```python
from build123d import *

# Parameters (mm, degrees)
SKETCH1_W            = 126
SKETCH1_H            = 96
SKETCH1_R            = 1.675
BOSS_EXTRUDE1_DEPTH  = 1
SKETCH2_W            = 5
SKETCH2_H            = 10
BOSS_EXTRUDE2_DEPTH  = 12
CUT_EXTRUDE1_REACH   = 134.578
SKETCH3_R            = 1.675
CUT_EXTRUDE2_START   = -2
CUT_EXTRUDE2_DEPTH   = 114.5
CHAMFER1_SIZE        = 2
CUT_EXTRUDE3_REACH   = 134.578
SKETCH5_R            = 1.675
CUT_EXTRUDE4_START   = -2
CUT_EXTRUDE4_DEPTH   = 114.5
SKETCH7_R            = 1.675
CUT_EXTRUDE5_DEPTH   = 10
SKETCH9_W            = 7
SKETCH9_H            = 28
CUT_EXTRUDE7_DEPTH   = 10
SKETCH11_R           = 1.675
SKETCH11_W           = 9
SKETCH11_H           = 6
CUT_EXTRUDE8_DEPTH   = 10
BOSS_EXTRUDE3_DEPTH  = 2
SKETCH24_W           = 19
SKETCH24_H           = 25.6
CUT_EXTRUDE17_DEPTH  = 2
FILLET1_R            = 2
SKETCH26_W           = 42.95
SKETCH26_H           = 12.988932873
SKETCH26_W_2         = 30.05
SKETCH26_H_2         = 41.011067127
SKETCH26_H_3         = 28
BOSS_EXTRUDE10_DEPTH = 3
FILLET2_R            = 2


with BuildPart() as part:
    # Sketch1 → Boss-Extrude1 (new body)
    with BuildSketch(Plane.XY):
        Rectangle(SKETCH1_W, SKETCH1_H)
        with Locations((53, 31)):
            Circle(SKETCH1_R, mode=Mode.SUBTRACT)
        with Locations((53, 21)):
            Circle(SKETCH1_R, mode=Mode.SUBTRACT)
    extrude(amount=BOSS_EXTRUDE1_DEPTH)

    # Sketch2 → Boss-Extrude2 (add)
    with BuildSketch(Plane(origin=(0, 0, 0), x_dir=(-1, 0, 0), z_dir=(0, 0, -1))):
        with Locations((-57.5, 40)):
            Rectangle(SKETCH2_W, SKETCH2_H)
        with Locations((57.5, 40)):
            Rectangle(SKETCH2_W, SKETCH2_H)
        with Locations((-57.5, -40)):
            Rectangle(SKETCH2_W, SKETCH2_H)
        with Locations((57.5, -40)):
            Rectangle(SKETCH2_W, SKETCH2_H)
    extrude(amount=BOSS_EXTRUDE2_DEPTH)

    # Cut-Extrude1: up to this face of the body (flat: up to its plane)
    cut_extrude1_end = Plane(part.part.faces().sort_by_distance((60, 40, -6))[0])
    # Sketch3 → Cut-Extrude1 (cut, up to the picked face)
    with BuildSketch(Plane.ZY.offset(60), mode=Mode.PRIVATE) as cut_extrude1_sk1:
        with Locations((-7, 40)):
            Circle(SKETCH3_R)
    cut_extrude1_tool1 = split(extrude(cut_extrude1_sk1.sketch, amount=-CUT_EXTRUDE1_REACH, mode=Mode.PRIVATE), bisect_by=cut_extrude1_end, keep=Keep.BOTH, mode=Mode.PRIVATE)
    add(cut_extrude1_tool1.solids().sort_by(Axis((-60, 40, -7), (1, 0, 0)))[0], mode=Mode.SUBTRACT)

    # Sketch4 → Cut-Extrude2 (cut)
    with BuildSketch(Plane(origin=(-55, 0, 0), x_dir=(0, 0, -1), z_dir=(1, 0, 0)).offset(CUT_EXTRUDE2_START)):
        Polygon((8.616580754, 42.8), (5.383419246, 42.8), (3.766838493, 40), (5.383419246, 37.2), (8.616580754, 37.2), (10.233161507, 40), align=None)
    extrude(amount=CUT_EXTRUDE2_DEPTH, mode=Mode.SUBTRACT)

    # Chamfer1
    chamfer1_edges = [part.edges().sort_by_distance(p)[0] for p in [
        (55, 40, 0),
        (-55, 40, 0),
        (55, -40, 0),
        (-55, -40, 0),
    ]]
    chamfer(chamfer1_edges, length=CHAMFER1_SIZE)

    # Cut-Extrude3: up to this face of the body (flat: up to its plane)
    cut_extrude3_end = Plane(part.part.faces().sort_by_distance((-60, -40, -6))[0])
    # Sketch5 → Cut-Extrude3 (cut, up to the picked face)
    with BuildSketch(Plane(origin=(60, 0, 0), x_dir=(0, 0, -1), z_dir=(1, 0, 0)), mode=Mode.PRIVATE) as cut_extrude3_sk1:
        with Locations((7, -40)):
            Circle(SKETCH5_R)
    cut_extrude3_tool1 = split(extrude(cut_extrude3_sk1.sketch, amount=-CUT_EXTRUDE3_REACH, mode=Mode.PRIVATE), bisect_by=cut_extrude3_end, keep=Keep.BOTH, mode=Mode.PRIVATE)
    add(cut_extrude3_tool1.solids().sort_by(Axis((60, -40, -7), (-1, 0, 0)))[0], mode=Mode.SUBTRACT)

    # Sketch6 → Cut-Extrude4 (cut)
    with BuildSketch(Plane(origin=(-55, 0, 0), x_dir=(0, 0, -1), z_dir=(1, 0, 0)).offset(CUT_EXTRUDE4_START)):
        Polygon((8.616580754, -37.2), (5.383419246, -37.2), (3.766838493, -40), (5.383419246, -42.8), (8.616580754, -42.8), (10.233161507, -40), align=None)
    extrude(amount=CUT_EXTRUDE4_DEPTH, mode=Mode.SUBTRACT)

    # Sketch7 → Cut-Extrude5 (cut)
    with BuildSketch(Plane.XY.offset(1)):
        with Locations((5.63, 30)):
            Circle(SKETCH7_R)
        with Locations((-2.37, 30)):
            Circle(SKETCH7_R)
    extrude(amount=-CUT_EXTRUDE5_DEPTH, mode=Mode.SUBTRACT)

    # Sketch9 → Cut-Extrude7 (cut)
    with BuildSketch(Plane.XY.offset(1)):
        with Locations((-9.87, 29)):
            Rectangle(SKETCH9_W, SKETCH9_H)
    extrude(amount=-CUT_EXTRUDE7_DEPTH, mode=Mode.SUBTRACT)

    # Sketch11 → Cut-Extrude8 (cut)
    with BuildSketch(Plane.XY.offset(1)):
        with Locations((22, -36.45)):
            Circle(SKETCH11_R)
        with Locations((22, -22.45)):
            Circle(SKETCH11_R)
        with Locations((-12.5, -23.2)):
            Rectangle(SKETCH11_W, SKETCH11_H)
    extrude(amount=-CUT_EXTRUDE8_DEPTH, mode=Mode.SUBTRACT)

    # Sketch21 → Boss-Extrude3 (add)
    # profile 1 of 4: a face of its own
    with BuildSketch(Plane(origin=(0, 0, 0), x_dir=(-1, 0, 0), z_dir=(0, 0, -1))):
        Polygon((-50.719466437, 24.95), (-55.280533563, 24.95), (-57.561067127, 21), (-55.280533563, 17.05), (-50.719466437, 17.05), (-48.438932873, 21), align=None)
        Polygon((-51.397853003, 23.775), (-54.602146997, 23.775), (-56.204293994, 21), (-54.602146997, 18.225), (-51.397853003, 18.225), (-49.795706006, 21), align=None, mode=Mode.SUBTRACT)
    # profile 2 of 4: a face of its own
    with BuildSketch(Plane(origin=(0, 0, 0), x_dir=(-1, 0, 0), z_dir=(0, 0, -1))):
        Polygon((-50.719466437, 34.95), (-55.280533563, 34.95), (-57.561067127, 31), (-55.280533563, 27.05), (-50.719466437, 27.05), (-48.438932873, 31), align=None)
        Polygon((-51.397853003, 33.775), (-54.602146997, 33.775), (-56.204293994, 31), (-54.602146997, 28.225), (-51.397853003, 28.225), (-49.795706006, 31), align=None, mode=Mode.SUBTRACT)
    # profile 3 of 4: a face of its own
    with BuildSketch(Plane(origin=(0, 0, 0), x_dir=(-1, 0, 0), z_dir=(0, 0, -1))):
        Polygon((6.32, 32.280533563), (2.37, 34.561067127), (-1.58, 32.280533563), (-1.58, 27.719466437), (2.37, 25.438932873), (6.32, 27.719466437), align=None)
        Polygon((5.145, 31.602146997), (2.37, 33.204293994), (-0.405, 31.602146997), (-0.405, 28.397853003), (2.37, 26.795706006), (5.145, 28.397853003), align=None, mode=Mode.SUBTRACT)
    # profile 4 of 4: a face of its own
    with BuildSketch(Plane(origin=(0, 0, 0), x_dir=(-1, 0, 0), z_dir=(0, 0, -1))):
        Polygon((-1.68, 32.280533563), (-5.63, 34.561067127), (-9.58, 32.280533563), (-9.58, 27.719466437), (-5.63, 25.438932873), (-1.68, 27.719466437), align=None)
        Polygon((-2.855, 31.602146997), (-5.63, 33.204293994), (-8.405, 31.602146997), (-8.405, 28.397853003), (-5.63, 26.795706006), (-2.855, 28.397853003), align=None, mode=Mode.SUBTRACT)
    extrude(amount=BOSS_EXTRUDE3_DEPTH)

    # Sketch24 → Cut-Extrude17 (cut)
    with BuildSketch(Plane.XY.offset(1)):
        with Locations((-46.7, 1.15)):
            Rectangle(SKETCH24_W, SKETCH24_H)
        Polygon((-37.2, 26.35), (-37.2, 13.95), (-37.2, -11.65), (-37.2, -24.05), (-33.8, -24.05), (-33.8, 26.35), align=None)
    extrude(amount=-CUT_EXTRUDE17_DEPTH, mode=Mode.SUBTRACT)

    # Fillet1
    fillet1_edges = [part.edges().sort_by_distance(p)[0] for p in [
        (57.5, 45, -12),
        (57.5, 35, -12),
        (-57.5, 45, -12),
        (-57.5, 35, -12),
        (57.5, -35, -12),
        (57.5, -45, -12),
        (-57.5, -35, -12),
        (-57.5, -45, -12),
    ]]
    fillet(fillet1_edges, radius=FILLET1_R)

    # Sketch26 → Boss-Extrude10 (add)
    with BuildSketch(Plane(origin=(0, 0, 0), x_dir=(-1, 0, 0), z_dir=(0, 0, -1))):
        Polygon((-27.95, -30.011067127), (-27.95, -43), (-55, -43), (-55, -45), (55, -45), (55, -43), (19, -43), (19, -30.011067127), (58, -30.011067127), (58, -35), (60, -35), (60, 35), (58, 35), (58, 32), (19, 32), (19, 43), (60, 43), (60, 45), (-60, 45), (-60, 43), (-27.95, 43), (-27.95, 15), (-58, 15), (-58, 35), (-60, 35), (-60, -35), (-58, -35), (-58, -30.011067127), align=None)
        with Locations((-4.475, -36.505533564)):
            Rectangle(SKETCH26_W, SKETCH26_H, mode=Mode.SUBTRACT)
        with Locations((-42.975, -7.505533564)):
            Rectangle(SKETCH26_W_2, SKETCH26_H_2, mode=Mode.SUBTRACT)
        with Locations((-4.475, -7.505533564)):
            Rectangle(SKETCH26_W, SKETCH26_H_2, mode=Mode.SUBTRACT)
        with Locations((-4.475, 29)):
            Rectangle(SKETCH26_W, SKETCH26_H_3, mode=Mode.SUBTRACT)
        Polygon((19, 15), (19, 30), (58, 30), (58, -28.011067127), (19, -28.011067127), (19, 13), (33.8, 13), (33.8, 15), align=None, mode=Mode.SUBTRACT)
    extrude(amount=BOSS_EXTRUDE10_DEPTH)

    # Fillet2
    fillet2_edges = [part.edges().sort_by_distance(p)[0] for p in [
        (-63, 48, 0.5),
        (63, 48, 0.5),
        (63, -48, 0.5),
        (-63, -48, 0.5),
    ]]
    fillet(fillet2_edges, radius=FILLET2_R)


solid = part.part
```
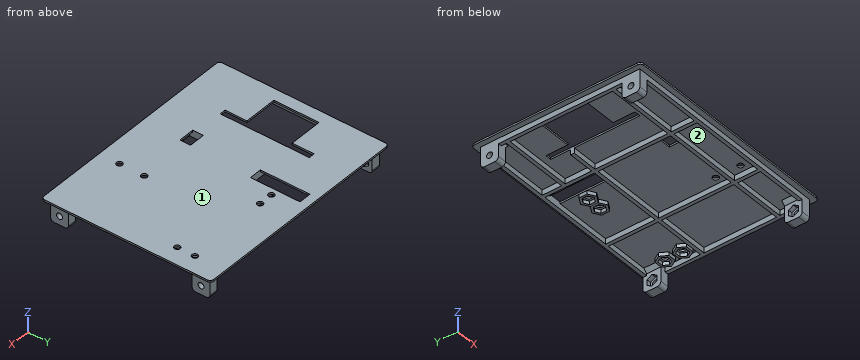
Verification items for the finished model (mm, model axes). Face numbers are marked on the shaded views. Coordinates: 2 decimals unless noted, no trailing zeros. Order: outer loops, then holes, each group sorted by start corner. A loop starts at its lowest first (then second) coordinate and runs counter-clockwise, first axis right, second up. Notation, with made-up numbers: (-31, 14) - (-6, 14) arc R21 ccw to (-6, 44) - close; hole circle Ø8 at (55.25, 26.25). An arc over 180 degrees is marked (long way). Return JSON: item names as keys, results as strings.
(1) Mould release check, pull along X, two halves, no side actions. Record for the marked faces 1 and 2: pulls with the +X half, pulls with the -X half, needs draft (parallel to the pull), parting line crosses it, or undercut.
Filled sheet:
{"face 1": "needs draft", "face 2": "undercut"}
(2) Go/stop test with flat-tipped pins: pin 1 (4.5 mm diameter, centred on x = -4.5, z = -1.5, fed in from +Y); pin 2 (2 mm diameter, centred on x = 53, z = -1.5, fed in from +Y); pin 3 (0.6 mm diameter, centred on y = 29.5, z = -1.5, fed in from -X); pin 4 (2.5 mm diameter, centred on x = -1, z = -1.5, fed in from -Y). Record where each tip stops, or that it passes through.
Filled sheet:
{"pin 1": "stops at y = 48", "pin 2": "stops at y = 45", "pin 3": "stops at x = -60", "pin 4": "stops at y = -45"}
(3) Section check D-D, the plane x = -26. Record the cut outline in (y, z), and give its area (3 significant figures).
Filled sheet:
{"outline": "(-48, 0) - (-45, 0) - (-45, -3) - (-43, -3) - (-43, 0) - (-30.01, 0) - (-30.01, -3) - (-28.01, -3) - (-28.01, 0) - (13, 0) - (13, -3) - (15, -3) - (15, 0) - (30, 0) - (30, -3) - (32, -3) - (32, 0) - (43, 0) - (43, -3) - (45, -3) - (45, 0) - (48, 0) - (48, 1) - (-48, 1) - close", "area": "126 mm^2"}
(4) Section check A-A, the plane x = -49. Record the cut outline in (y, z).
Filled sheet:
{"outline": "(-48, 0) - (-45, 0) - (-45, -3) - (-43, -3) - (-43, 0) - (-30.01, 0) - (-30.01, -3) - (-28.01, -3) - (-28.01, 0) - (-11.65, 0) - (-11.65, 1) - (-48, 1) - close; (13.95, 0) - (30, 0) - (30, -3) - (32, -3) - (32, 0) - (43, 0) - (43, -3) - (45, -3) - (45, 0) - (48, 0) - (48, 1) - (13.95, 1) - close"}
(5) Section check B-B, the plane y = 11. Record the cut outline in (x, z), and give its area (3 significant figures).
Filled sheet:
{"outline": "(-63, 0) - (-60, 0) - (-60, -3) - (-58, -3) - (-58, 0) - (-56.2, 0) - (-56.2, 1) - (-63, 1) - close; (-33.8, 0) - (-19, 0) - (-19, -3) - (-17, -3) - (-17, 0) - (25.95, 0) - (25.95, -3) - (27.95, -3) - (27.95, 0) - (58, 0) - (58, -3) - (60, -3) - (60, 0) - (63, 0) - (63, 1) - (-33.8, 1) - close", "area": "128 mm^2"}
(6) Thickness scan on line 1 along Y through (x, z) = (22, 0.7) (3 decimals); line 2 along Y through (x, z) = (58.05, -7) (3 decimals); line 3 along X through (y, z) = (36.5, -6.5). Record the ranges inside material, lowest first.
Filled sheet:
{"line 1": "y = -48 to -38.125, -34.775 to -24.125, -20.775 to 48", "line 2": "y = -45 to -41.675, -38.325 to -35, 35 to 38.325, 41.675 to 45", "line 3": "x = -60 to -55, 55 to 60"}
(7) Section check C-C, the plane x = 22. Record the cut outline in (y, z) (3 decimals), and give its area (3 significant figures).
Filled sheet:
{"outline": "(-48, 0) - (-45, 0) - (-45, -3) - (-43, -3) - (-43, 0) - (-38.125, 0) - (-38.125, 1) - (-48, 1) - close; (-34.775, 0) - (-30.011, 0) - (-30.011, -3) - (-28.011, -3) - (-28.011, 0) - (-24.125, 0) - (-24.125, 1) - (-34.775, 1) - close; (-20.775, 0) - (13, 0) - (13, -3) - (15, -3) - (15, 0) - (43, 0) - (43, -3) - (45, -3) - (45, 0) - (48, 0) - (48, 1) - (-20.775, 1) - close", "area": "113 mm^2"}
